```python
from build123d import *

# Parameters (mm, degrees)
SKETCH1_W               = 212
SKETCH1_H               = 70
BOSS_EXTRUDE1_DEPTH     = 3
SKETCH2_W               = 6
SKETCH2_H               = 50
CUT_EXTRUDE1_DEPTH      = 1
CUT_EXTRUDE1_DEPTH_BACK = 4
FILLET1_R               = 10


with BuildPart() as part:
    # Sketch1 → Boss-Extrude1 (new body)
    with BuildSketch(Plane(origin=(0, 0, 0), x_dir=(1, 0, 0), z_dir=(0, 1, 0))):
        Rectangle(SKETCH1_W, SKETCH1_H)
    extrude(amount=BOSS_EXTRUDE1_DEPTH)

    # Sketch2 → Cut-Extrude1 (cut, two sides)
    with BuildSketch(Plane(origin=(0, 3, 0), x_dir=(1, 0, 0), z_dir=(0, 1, 0))) as cut_extrude1_sk:
        with Locations((23, 0)):
            Rectangle(SKETCH2_W, SKETCH2_H)
        with Locations((-93, 0)):
            Rectangle(SKETCH2_W, SKETCH2_H)
        with Locations((37, 0)):
            Rectangle(SKETCH2_W, SKETCH2_H)
        with Locations((93, 0)):
            Rectangle(SKETCH2_W, SKETCH2_H)
    extrude(amount=CUT_EXTRUDE1_DEPTH, mode=Mode.SUBTRACT)
    extrude(cut_extrude1_sk.sketch, amount=-CUT_EXTRUDE1_DEPTH_BACK, mode=Mode.SUBTRACT)

    # Fillet1
    fillet1_edges = [part.edges().sort_by_distance(p)[0] for p in [
        (106, 1.5, 35),
        (-106, 1.5, 35),
        (-106, 1.5, -35),
        (106, 1.5, -35),
    ]]
    fillet(fillet1_edges, radius=FILLET1_R)


solid = part.part
```
CAD build for the part. Positions are in the model's coordinates, mm. Coordinates: 2 decimals unless noted, no trailing zeros. Order: outer loops, then holes, each group sorted by start corner. A loop starts at its lowest first (then second) coordinate and runs counter-clockwise, first axis right, second up. Notation, with made-up numbers: M -36.5,79.5 L -0.5,79.5 A33 ccw -0.5,107.5 Z; hole C -2,-40 d4. An arc over 180 degrees is marked long. Write each question's results on one line, items separated by ' | '. Start each with the question number.
Q1. Cut at A-A (x = 38). List the corners of the cut face in (y, z).
Q2. Drill centre lines: probe 1 along X at (y, z) = (0.5, -12); probe 2 along Z at (x, y) = (36, 2.1); probe 3 along Z at (x, y) = (-96.5, 1.9). Where is each one in solid material? Low to high. Write a range as from..to.
Q3. Cut at B-B (z = 18.5). List the corners of the cut face in (x, y), then the cut area to 3 significant figures.
Q4. Cut at C-C (y = 1.5). List the corners of the cut face in (x, z), then the cut area to 3 significant figures.
Found:
1) outline: M 0,-35 L 3,-35 L 3,-25 L 0,-25 Z; M 0,25 L 3,25 L 3,35 L 0,35 Z
2) probe 1: -106..-96, -90..20, 26..34, 40..90, 96..106 | probe 2: -35..-25, 25..35 | probe 3: -34.99..34.99
3) outline: M -106,0 L -96,0 L -96,3 L -106,3 Z; M -90,0 L 20,0 L 20,3 L -90,3 Z; M 26,0 L 34,0 L 34,3 L 26,3 Z; M 40,0 L 90,0 L 90,3 L 40,3 Z; M 96,0 L 106,0 L 106,3 L 96,3 Z | area: 564 mm²
4) outline: M -106,-25 A10 ccw -96,-35 L 96,-35 A10 ccw 106,-25 L 106,25 A10 ccw 96,35 L -96,35 A10 ccw -106,25 Z; hole M -96,-25 L -90,-25 L -90,25 L -96,25 Z; hole M 20,-25 L 26,-25 L 26,25 L 20,25 Z; hole M 34,-25 L 40,-25 L 40,25 L 34,25 Z; hole M 90,-25 L 96,-25 L 96,25 L 90,25 Z | area: 13,600 mm²
